```python
from build123d import *

# Parameters (mm, degrees)
BASE_FLANGE1_DEPTH = 11
FILLET1_R          = 5
SKETCH6_R          = 2.75
CUT_EXTRUDE1_DEPTH = 10


# Sheet-metal steps are written as plain solids
with BuildPart() as part:
    # Sketch1 → Base-Flange1 (new body)
    with BuildSketch(Plane.XY):
        with BuildLine():
            Line((-12.8, 0), (-12.8, 3.7))
            ThreePointArc((-12.8, 3.7), (-13.385786438, 5.114213562), (-14.8, 5.7))
            Line((-14.8, 5.7), (-25.3, 5.7))
            Line((-25.3, 5.7), (-25.3, 5.2))
            Line((-25.3, 5.2), (-15.3, 5.2))
            ThreePointArc((-15.3, 5.2), (-13.885786438, 4.614213562), (-13.3, 3.2))
            Line((-13.3, 3.2), (-13.3, 0))
            ThreePointArc((-13.3, 0), (0, -13.3), (13.3, 0))
            Line((13.3, 0), (13.3, 3.2))
            ThreePointArc((13.3, 3.2), (13.885786438, 4.614213562), (15.3, 5.2))
            Line((15.3, 5.2), (25.3, 5.2))
            Line((25.3, 5.2), (25.3, 5.7))
            Line((25.3, 5.7), (14.8, 5.7))
            ThreePointArc((14.8, 5.7), (13.385786438, 5.114213562), (12.8, 3.7))
            Line((12.8, 3.7), (12.8, 0))
            ThreePointArc((12.8, 0), (0, -12.8), (-12.8, 0))
        make_face()
    extrude(amount=-BASE_FLANGE1_DEPTH)

    # Fillet1
    fillet1_edges = [part.edges().sort_by_distance(p)[0] for p in [
        (25.3, 5.45, 0),
        (-25.3, 5.45, 0),
        (-25.3, 5.45, -11),
        (25.3, 5.45, -11),
    ]]
    fillet(fillet1_edges, radius=FILLET1_R)

    # Sketch6 → Cut-Extrude1 (cut)
    with BuildSketch(Plane(origin=(0, 0, 0), x_dir=(1, 0, 0), z_dir=(0, 1, 0))):
        with Locations((19.35, 5.5)):
            Circle(SKETCH6_R)
        with Locations((-19.35, 5.5)):
            Circle(SKETCH6_R)
    extrude(amount=CUT_EXTRUDE1_DEPTH, mode=Mode.SUBTRACT)


solid = part.part
```
CAD build for the part. Positions are in the model's coordinates, mm. A direction names the side the tool comes from. Round coordinates to 2 decimals unless told otherwise and drop trailing zeros. Order: outer loops, then holes, each group sorted by start corner. A loop starts at its lowest first (then second) coordinate and runs counter-clockwise, first axis right, second up.
Item 1: Tool access for faces 4 (the face through (22.5, 5.2, -5.4)), 5 (the face through (-23, 5.2, -5)), 6 (the face through (23.87, 5.45, -9.5)), 7 (the face through (-13.37, 5.1, -5.42)): list every direction of +Z, -Z, +X, -X, +Y, -Y with a clear straight run to the whole face (end or side of a thin tool).
Item 2: Saw through at B-B on z = -5.5. Write the cut outline in (x, y).
Item 3: Pin check, flat tips, straight feed: pin 1 (5 mm diameter, centred on x = 21.5, z = -5, fed in from -Y); pin 2 (3.5 mm diameter, centred on x = -19.35, z = -5.5, fed in from +Y); pin 3 (6 mm diameter, centred on y = -1.5, z = -2.5, fed in from +X); pin 4 (1.5 mm diameter, centred on x = 12.5, z = -9, fed in from -Y). Stop position of each tip, or through.
Item 4: Saw through at D-D on z = -7.75. Write the cut outline in (x, y), then the cut area to 3 significant figures.
Item 5: Mould opens along Z. For faces 1 (the face through (0, -13, -11)), 2 (the face through (-21.532, 5.446, -3.827)), 3 (the face through (-23.87, 5.45, -1.5)) say: pulls with the +Z half, pulls with the -Z half, needs draft (parallel to the pull), parting line crosses it, or undercut.
Item 6: Saw through at C-C on y = -11. Write the cut outline in (x, z).
Item 7: Saw through at A-A on x = -19.35. Write the cut outline in (y, z).
Item 8: Probe line 1 along Z through (x, y) = (-19.35, 5.55); line 2 along X through (y, z) = (1.25, -4.25); line 3 along Y through (x, z) = (0.5, -2.5). List the from-to ranges inside material, lowest first.
Reported:
1. face 4: +Z, -Z, +X, -Y
1. face 5: +Z, -Z, -X, -Y
1. face 6: -Z, +X, +Y, -Y
1. face 7: +Z, -Z, +Y
2. outline: (-25.3, 5.2) - (-22.1, 5.2) - (-22.1, 5.7) - (-25.3, 5.7) - close; (-16.6, 5.2) - (-15.3, 5.2) arc R2 cw to (-13.3, 3.2) - (-13.3, 0) arc R13.3 ccw to (13.3, 0) - (13.3, 3.2) arc R2 cw to (15.3, 5.2) - (16.6, 5.2) - (16.6, 5.7) - (14.8, 5.7) arc R2 ccw to (12.8, 3.7) - (12.8, 0) arc R12.8 cw to (-12.8, 0) - (-12.8, 3.7) arc R2 ccw to (-14.8, 5.7) - (-16.6, 5.7) - close; (22.1, 5.2) - (25.3, 5.2) - (25.3, 5.7) - (22.1, 5.7) - close
3. pin 1: stops at y = 5.2
3. pin 2: passes through
3. pin 3: stops at x = 13.3
3. pin 4: stops at y = -6.23
4. outline: (-24.98, 5.2) - (-20.93, 5.2) - (-20.93, 5.7) - (-24.98, 5.7) - close; (-17.77, 5.2) - (-15.3, 5.2) arc R2 cw to (-13.3, 3.2) - (-13.3, 0) arc R13.3 ccw to (13.3, 0) - (13.3, 3.2) arc R2 cw to (15.3, 5.2) - (17.77, 5.2) - (17.77, 5.7) - (14.8, 5.7) arc R2 ccw to (12.8, 3.7) - (12.8, 0) arc R12.8 cw to (-12.8, 0) - (-12.8, 3.7) arc R2 ccw to (-14.8, 5.7) - (-17.77, 5.7) - close; (20.93, 5.2) - (24.98, 5.2) - (24.98, 5.7) - (20.93, 5.7) - close
4. area: 34.7 mm2
5. face 1: pulls with the -Z half
5. face 2: undercut
5. face 3: pulls with the +Z half
6. outline: (-7.48, -11) - (-6.55, -11) - (-6.55, 0) - (-7.48, 0) - close; (6.55, -11) - (7.48, -11) - (7.48, 0) - (6.55, 0) - close
7. outline: (5.2, -11) - (5.7, -11) - (5.7, -8.25) - (5.2, -8.25) - close; (5.2, -2.75) - (5.7, -2.75) - (5.7, 0) - (5.2, 0) - close
8. line 1: z = -11 to -8.25, -2.75 to 0
8. line 2: x = -13.3 to -12.8, 12.8 to 13.3
8. line 3: y = -13.29 to -12.79
